CAD build for the part. Positions are in the model's coordinates, mm. Face numbers are marked on the shaded views. A direction names the side the tool comes from. Coordinates: 2 decimals unless noted, no trailing zeros. Loops run counter-clockwise (first coordinate to the right, second up) from the corner with the lowest first, then second, coordinate; pieces in that order, holes last. Notation, with made-up numbers: (46, -1.75) -> (88, -1.75) arc R16 cw to (88, 4.25) -> close; hole circle Ø1 at (-21, 48.25). An arc over 180 degrees is marked (long way). Return JSON: item names as keys, results as strings. Group by question number.
(1) Saw through at B-B on x = 35. Write the cut outline in (y, z), then the cut area to 3 significant figures.
(2) Saw through at D-D on y = 4.3. Give the number of separate pieces and of enclosed holes in the cut face, then the cut area to 3 significant figures.
(3) Saw through at C-C on z = 23.5. Write the cut outline in (x, y), then the cut area to 3 significant figures.
(4) Probe L1, parallel to X at y = 3.85, z = 12.5; L2, parallel to Z at x = 11, y = 1.55; L3, parallel to X at y = 4.65, z = 23. List the from-to ranges inside material, lowest first.
(5) Tool access for the marked faces 4, 5, 6, 7 and 8: list every direction of +Z, -Z, +X, -X, +Y, -Y with a clear straight run to the whole face (end or side of a thin tool).
(6) Flat gauge pins, fed straight in: pin 1 Ø1.2 at (y, z) = (3.5, 26.5) entering from -X; pin 2 Ø3.5 at (x, y) = (1, 3) entering from -Z; pin 3 Ø2 at (x, z) = (17.5, 12.5) entering from +Y. Where does each tip first touch, or does it go through?
(7) Mould opens along Z. For the marked faces 1, 2 and 3 say: pulls with the +Z half, pulls with the -Z half, needs draft (parallel to the pull), parting line crosses it, or undercut.
(8) Saw through at A-A on z = 12.5. Write the cut outline in (x, y), then the cut area to 3 significant figures.
```python
from build123d import *

# Parameters (mm, degrees)
SKETCH_1_R      = 1.25
SKETCH_1_R_2    = 3
EXTRUDE_1_DEPTH = 6


with BuildPart() as part:
    # 草图1 → 凸台-拉伸1 (new body)
    with BuildSketch(Plane(origin=(0, 0, 0), x_dir=(1, 0, 0), z_dir=(0, 1, 0))):
        Polygon((35.5, -24), (34.25, -24), (34.25, -20), (35.5, -20), (35.5, -18), (38.5, -18), (38.5, -20), (39.75, -20), (39.75, -24), (38.5, -24), (38.5, -28), (47, -28), (47, -25), (50, -25), (50, 0), (47, 0), (47, 3), (38.5, 3), (38.5, -1), (39.75, -1), (39.75, -5), (38.5, -5), (38.5, -7), (35.5, -7), (35.5, -5), (34.25, -5), (34.25, -1), (35.5, -1), (35.5, 3), (27, 3), (27, 0), (23, 0), (23, 3), (14.5, 3), (14.5, -1), (15.75, -1), (15.75, -5), (14.5, -5), (14.5, -7), (11.5, -7), (11.5, -5), (10.25, -5), (10.25, -1), (11.5, -1), (11.5, 3), (3, 3), (3, 0), (0, 0), (0, -25), (3, -25), (3, -28), (11.5, -28), (11.5, -24), (10.25, -24), (10.25, -20), (11.5, -20), (11.5, -18), (14.5, -18), (14.5, -20), (15.75, -20), (15.75, -24), (14.5, -24), (14.5, -28), (23, -28), (23, -25), (27, -25), (27, -28), (35.5, -28), align=None)
        with Locations(Location((32.5, -12.5, 0), (0, 0, 270))):
            Circle(SKETCH_1_R, mode=Mode.SUBTRACT)
        with Locations(Location((25, -12.5, 0), (0, 0, 270))):
            Circle(SKETCH_1_R_2, mode=Mode.SUBTRACT)
        with Locations(Location((17.5, -12.5, 0), (0, 0, 270))):
            Circle(SKETCH_1_R, mode=Mode.SUBTRACT)
        with Locations(Location((25, -20, 0), (0, 0, 270))):
            Circle(SKETCH_1_R, mode=Mode.SUBTRACT)
        with Locations(Location((25, -5, 0), (0, 0, 270))):
            Circle(SKETCH_1_R, mode=Mode.SUBTRACT)
    extrude(amount=EXTRUDE_1_DEPTH)


solid = part.part
```
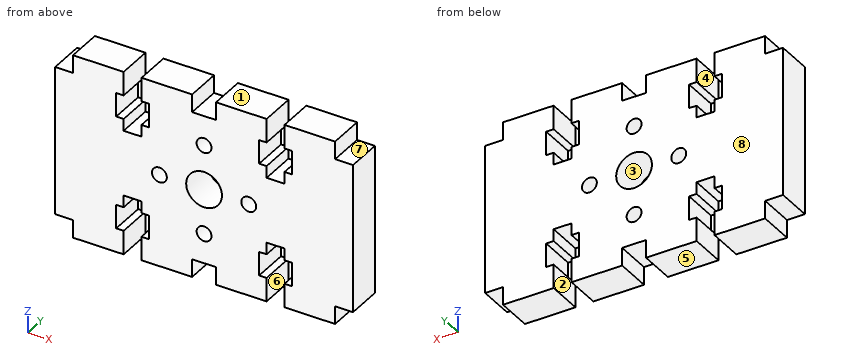
Geometry results:
{
 "1": {"outline": "(0, -3) -> (6, -3) -> (6, 1) -> (0, 1) -> close; (0, 5) -> (6, 5) -> (6, 20) -> (0, 20) -> close; (0, 24) -> (6, 24) -> (6, 28) -> (0, 28) -> close", "area": "138 mm²"},
 "2": {"separate pieces": "1", "enclosed holes": "5", "area": "1,280 mm²"},
 "3": {"outline": "(0, 0) -> (10.25, 0) -> (10.25, 6) -> (0, 6) -> close; (15.75, 0) -> (34.25, 0) -> (34.25, 6) -> (15.75, 6) -> close; (39.75, 0) -> (50, 0) -> (50, 6) -> (39.75, 6) -> close", "area": "234 mm²"},
 "4": {"L1": "0 to 16.25, 18.75 to 22, 28 to 31.25, 33.75 to 50", "L2": "-3 to 1, 5 to 20, 24 to 28", "L3": "0 to 10.25, 15.75 to 34.25, 39.75 to 50"},
 "5": {"face 4": "+Z, +Y, -Y", "face 5": "-Z, +X, -X, +Y, -Y", "face 6": "-Z, +Y, -Y", "face 7": "+Z, +X, +Y, -Y", "face 8": "+Z, -Z, +X, -X, +Y"},
 "6": {"pin 1": "x = 3", "pin 2": "z = 0", "pin 3": "through"},
 "7": {"face 1": "pulls with the +Z half", "face 2": "needs draft", "face 3": "undercut"},
 "8": {"outline": "(0, 0) -> (16.25, 0) -> (16.25, 6) -> (0, 6) -> close; (18.75, 0) -> (22, 0) -> (22, 6) -> (18.75, 6) -> close; (28, 0) -> (31.25, 0) -> (31.25, 6) -> (28, 6) -> close; (33.75, 0) -> (50, 0) -> (50, 6) -> (33.75, 6) -> close", "area": "234 mm²"}
}
